The listing builds one solid part. Answer for the finished solid, in the listing's coordinates (mm). A direction names the side the tool comes from. Round coordinates to 2 decimals unless told otherwise and drop trailing zeros. Write each loop counter-clockwise with the first axis right and the second up, starting at its lowest first coordinate (ties: lowest second). Pieces come first, ordered by that corner, then holes. Notation, with made-up numbers: (-22.5, 55) - (6.5, 55) arc R23 cw to (6.5, 63) - close; hole circle Ø1 at (62, -30). An arc over 180 degrees is marked (long way). Answer as CSV lines item,"result". Start each with the question number.
Item 1: A cutting plane is placed at C-C on y = 4. Determine the outline of the cut face in (x, z), and give its area (3 significant figures).
Item 2: Straight lines are drawn through the part: line 1 along X through (y, z) = (2.1, 0); line 2 along Y through (x, z) = (-4, 4.75). For each, find the intervals that lie inside material, in ascending order. Write a range as [from, to].
Item 3: For a pull along Z with two mould halves and no side action, classify faces 1 (the flat face through (3, 6.9, -3)), 2 (the cylindrical face through (-0.388, 2.991, -2.955)), 3 (the cylindrical face through (-1.02, 2.42, 4.59)) as pulls with the +Z half, pulls with the -Z half, needs draft (parallel to the pull), parting line crosses it, or undercut.
Item 4: Flat-ended cylindrical pins translate along their axes: pin 1 (6 mm diameter, centred on x = -5.5, z = -4, fed in from +Y); pin 2 (4 mm diameter, centred on x = -5.5, y = 5.5, fed in from -Z); pin 3 (4 mm diameter, centred on y = 2.5, z = -5.5, fed in from -X). Find the tip coordinate at first contact, or state that the pin passes through.
Item 5: A cutting plane is placed at B-B on x = 0. Determine the outline of the cut face in (y, z), and give its area (3 significant figures).
Item 6: Which of the six approach directions +Z, -Z, +X, -X, +Y, -Y give full straight-line access (tool end or side, diameter ignored) to faces 4 (the cylindrical face through (-7.493, 5.393, -0.33)), 5 (the flat face through (0, 4.9, 5))?
Item 7: A cutting plane is placed at A-A on z = 0. Determine the outline of the cut face in (x, y), and give its area (3 significant figures).
```python
from build123d import *

# Parameters (mm, degrees)
SKETCH1_R           = 4.7
BOSS_EXTRUDE1_DEPTH = 4.9
SKETCH2_R           = 7.5
BOSS_EXTRUDE2_DEPTH = 2
SKETCH3_R           = 2.98
CUT_EXTRUDE1_DEPTH  = 7.9
CHAMFER1_SIZE       = 1
CHAMFER2_SIZE       = 1


with BuildPart() as part:
    # Sketch1 → Boss-Extrude1 (new body)
    with BuildSketch(Plane(origin=(0, 0, 0), x_dir=(1, 0, 0), z_dir=(0, 1, 0))):
        Circle(SKETCH1_R)
    extrude(amount=BOSS_EXTRUDE1_DEPTH)

    # Sketch2 → Boss-Extrude2 (add)
    with BuildSketch(Plane(origin=(0, 4.9, 0), x_dir=(1, 0, 0), z_dir=(0, 1, 0))):
        Circle(SKETCH2_R)
    extrude(amount=BOSS_EXTRUDE2_DEPTH)

    # Sketch3 → Cut-Extrude1 (cut, through all)
    with BuildSketch(Plane(origin=(0, 6.9, 0), x_dir=(1, 0, 0), z_dir=(0, 1, 0))):
        Circle(SKETCH3_R)
    extrude(amount=-CUT_EXTRUDE1_DEPTH, mode=Mode.SUBTRACT)

    # Chamfer1
    chamfer1_edges = [part.edges().sort_by_distance(p)[0] for p in [
        (-2.98, 6.9, 0),
    ]]
    chamfer(chamfer1_edges, length=CHAMFER1_SIZE)

    # Chamfer2
    chamfer2_edges = [part.edges().sort_by_distance(p)[0] for p in [
        (-7.5, 6.9, 0),
    ]]
    chamfer(chamfer2_edges, length=CHAMFER2_SIZE)


solid = part.part
```
Geometry says:
1,outline,"circle Ø9.4 at (0, 0); hole circle Ø5.96 at (0, 0)"
1,area,"41.5 mm^2"
2,line 1,"x = [-4.7, -2.98], [2.98, 4.7]"
2,line 2,"y = [4.9, 6.9]"
3,face 1,"needs draft"
3,face 2,"undercut"
3,face 3,"parting line crosses it"
4,pin 1,"stops at y = 6.9"
4,pin 2,"stops at z = -6.63"
4,pin 3,"stops at x = -3.14"
5,outline,"(0, -4.7) - (4.9, -4.7) - (4.9, -7.5) - (5.9, -7.5) - (6.9, -6.5) - (6.9, -3.98) - (5.9, -2.98) - (0, -2.98) - close; (0, 2.98) - (5.9, 2.98) - (6.9, 3.98) - (6.9, 6.5) - (5.9, 7.5) - (4.9, 7.5) - (4.9, 4.7) - (0, 4.7) - close"
5,area,"32.9 mm^2"
6,face 4,"+Y, -Y"
6,face 5,"-Y"
7,outline,"(-7.5, 4.9) - (-4.7, 4.9) - (-4.7, 0) - (-2.98, 0) - (-2.98, 5.9) - (-3.98, 6.9) - (-6.5, 6.9) - (-7.5, 5.9) - close; (2.98, 0) - (4.7, 0) - (4.7, 4.9) - (7.5, 4.9) - (7.5, 5.9) - (6.5, 6.9) - (3.98, 6.9) - (2.98, 5.9) - close"
7,area,"32.9 mm^2"
